Geometry: final body of the model. Coordinates: model frame, mm. Face numbers are marked on the shaded views. A direction names the side the tool comes from. Round coordinates to 2 decimals unless told otherwise and drop trailing zeros. Order: outer loops, then holes, each group sorted by start corner. A loop starts at its lowest first (then second) coordinate and runs counter-clockwise, first axis right, second up. Notation, with made-up numbers: M 55.5,-34 L 64.5,-34 A24 cw 64.5,-23 Z; hole C 52,42.25 d6. An arc over 180 degrees is marked long. Put each result on its own line as item: value. Start each with the question number.
1) Draft query along Y for the marked faces 1, 2 and 3. Return one class per face: pulls with the +Y half, pulls with the -Y half, needs draft (parallel to the pull), parting line crosses it, or undercut.
2) Access query for the marked faces 4, 5, 6 and 7. Directions: +Z, -Z, +X, -X, +Y, -Y. A direction counts if a zero-diameter tool reaches every point of the face in a straight line with its end or side. Return the directions, or none.
3) Section C-C, the plane x = 16.5. Return loops of the section in (y, z), then the cut area to 3 significant figures.
4) Section A-A, the plane x = 5. Return loops of the section in (y, z).
5) Section D-D, the plane y = 6.25. Return loops of the section in (x, z), then the cut area to 3 significant figures.
6) Material intervals for probe 1 along Y at (x, z) = (42, -17); probe 2 along X at (y, z) = (-0.25, 15); probe 3 along X at (y, z) = (-4.5, 5), sorted ascending. Write a range as [from, to].
7) First-contact query: P1, Ø6, axis at x = 42, y = 0, coming from the -Z side; P2, Ø3, axis at y = 5, z = 14, coming from the +X side; P3, Ø3, axis at x = 5, y = 0, coming from the -Z side; P4, Ø8, axis at y = 4.5, z = 16, coming from the -X side. Flat tips, straight axial feed; report the tip coordinate or a pass-through.
8) Section B-B, the plane z = 2. Return loops of the section in (x, y), then the cut area to 3 significant figures.
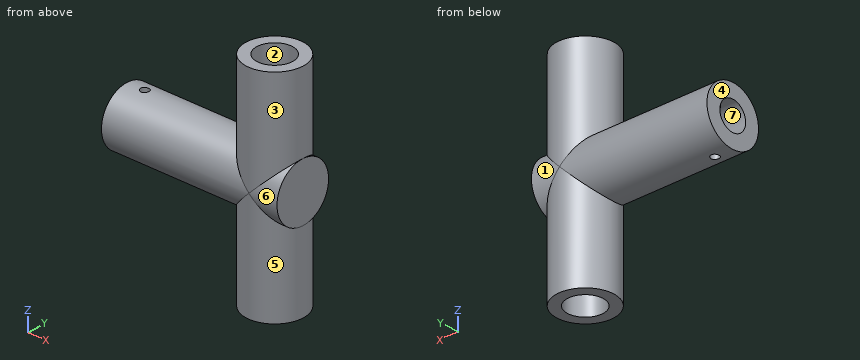
from build123d import *

# Parameters (mm, degrees)
SKETCH_2_R               = 8
EXTRUDE_1_DEPTH          = 50
SKETCH_3_R               = 4
CUT_EXTRUDE_1_DEPTH      = 40
SKETCH_4_R               = 1.15
CUT_EXTRUDE_2_DEPTH      = 9
CUT_EXTRUDE_2_DEPTH_BACK = 9
SKETCH_5_R               = 8
EXTRUDE_2_DEPTH          = 30
EXTRUDE_2_DEPTH_BACK     = 30
SKETCH_6_R               = 5
CUT_EXTRUDE_4_DEPTH      = 61


with BuildPart() as part:
    # 草图2 → 凸台-拉伸1 (new body)
    with BuildSketch(Plane(origin=(0, 0, 0), x_dir=(0, 0, -1), z_dir=(1, 0, 0))):
        Circle(SKETCH_2_R)
    extrude(amount=EXTRUDE_1_DEPTH)

    # 草图3 → 切除-拉伸1 (cut)
    with BuildSketch(Plane.ZY):
        Circle(SKETCH_3_R)
    extrude(amount=-CUT_EXTRUDE_1_DEPTH, mode=Mode.SUBTRACT)

    # 草图4 → 切除-拉伸2 (cut, two sides)
    with BuildSketch(Plane.XY) as cut_extrude_2_sk:
        with Locations((5, 0)):
            Circle(SKETCH_4_R)
    extrude(amount=CUT_EXTRUDE_2_DEPTH, mode=Mode.SUBTRACT)
    extrude(cut_extrude_2_sk.sketch, amount=-CUT_EXTRUDE_2_DEPTH_BACK, mode=Mode.SUBTRACT)

    # 草图5 → 凸台-拉伸2 (add, two sides)
    with BuildSketch(Plane.XY) as extrude_2_sk:
        with Locations((42, 0)):
            Circle(SKETCH_5_R)
    extrude(amount=EXTRUDE_2_DEPTH)
    extrude(extrude_2_sk.sketch, amount=-EXTRUDE_2_DEPTH_BACK)

    # 草图6 → 切除-拉伸4 (cut, through all)
    with BuildSketch(Plane(origin=(0, 0, -30), x_dir=(-1, 0, 0), z_dir=(0, 0, -1))):
        with Locations((-42, 0)):
            Circle(SKETCH_6_R)
    extrude(amount=-CUT_EXTRUDE_4_DEPTH, mode=Mode.SUBTRACT)


solid = part.part
Result sheet:
1. face 1: pulls with the +Y half
1. face 2: undercut
1. face 3: parting line crosses it
2. face 4: +Z, -Z, -X, +Y, -Y
2. face 5: -Z
2. face 6: +X, -Y
2. face 7: -X
3. outline: C 0,0 d16; hole C 0,0 d8
3. area: 151 mm2
4. outline: M -1.15,-7.92 L -1.15,-3.83 A4 cw -1.15,3.83 L -1.15,7.92 A8 ccw Z; M 1.15,-7.92 A8 ccw 1.15,7.92 L 1.15,3.83 A4 cw 1.15,-3.83 Z
5. outline: M 0,-4.99 L 37.01,-4.99 L 37.01,-30 L 46.99,-30 L 46.99,-4.99 L 50,-4.99 L 50,4.99 L 46.99,4.99 L 46.99,30 L 37.01,30 L 37.01,4.99 L 0,4.99 Z
5. area: 999 mm2
6. probe 1: y = [-8, -5], [5, 8]
6. probe 2: x = [34, 37.01], [46.99, 50]
6. probe 3: x = [0, 39.82], [44.18, 50]
7. P1: passes through
7. P2: stops at x = 49.19
7. P3: stops at z = -8
7. P4: stops at x = 34.02
8. outline: M 0,-7.75 L 40,-7.75 A8 ccw 44,-7.75 L 50,-7.75 L 50,7.75 L 44,7.75 A8 ccw 40,7.75 L 0,7.75 L 0,3.46 L 34.79,3.46 A8 ccw 34.79,-3.46 L 0,-3.46 Z; hole C 42,0 d10
8. area: 460 mm2
